Here's how the part is built. I have some questions about the finished solid (model axes, mm). Face numbers are marked on the shaded views. A direction names the side the tool comes from. Give positions to 0.01 mm unless a question says otherwise; leave off trailing zeros. Write each loop counter-clockwise with the first axis right and the second up, starting at its lowest first coordinate (ties: lowest second). Pieces come first, ordered by that corner, then holes. Notation, with made-up numbers: (68, -5.75) -> (83, -5.75) arc R17 cw to (83, 1.25) -> close; hole circle Ø8 at (11, 80). An arc over 180 degrees is marked (long way). Use CSV: the item, a comma, the result in double quotes. Start each with the question number.
(1) For pin 1 Ø1.5 at (x, y) = (12.5, 9.5) entering from -Z; pin 2 Ø5 at (x, z) = (16.8, -5) entering from -Y; pin 3 Ø2.5 at (x, y) = (4.8, 8.6) entering from -Z, each with a flat end and sliding along its axis, tell me the tip position at first contact or that it passes through.
(2) If we mould it in two halves opening along X, with no side actions, what happens to the marked faces 1, 2 and 3? For each: pulls with the +X half, pulls with the -X half, needs draft (parallel to the pull), parting line crosses it, or undercut.
(3) Suppose I cut it at D-D on x = 10.5. List the corners of the cut face in (y, z) for me, plus the area to 3 significant figures.
(4) Suppose I cut it at C-C on x = 4.8. List the corners of the cut face in (y, z) for me, plus the area to 3 significant figures.
(5) I need wall thicknesses on L1, parallel to Y at x = 4.8, z = 1.05; L2, parallel to Z at x = 1.5, y = 9.75; L3, parallel to Z at x = 16.8, y = 13.45. Which ranges of each line are inside material? Lowest first, please. Write a range as [from, to].
(6) Suppose I cut it at B-B on y = 8.6. List the corners of the cut face in (x, z) for me.
(7) Suppose I cut it at A-A on z = -5. List the corners of the cut face in (x, y) for me.
(8) Which directions (+Z, -Z, +X, -X, +Y, -Y) give clear straight access to the entire face, cutting with the end or side of a thin tool? Please do the marked faces 4 and 5.
from build123d import *

# Parameters (mm, degrees)
SKETCH_W     = 19.8
SKETCH_H     = 14.5
SKETCH_R     = 1.5
PAD_DEPTH    = 3
SKETCH001_W  = 19.8
SKETCH001_H  = 3
PAD001_DEPTH = 10
SKETCH002_R  = 1.5
POCKET_DEPTH = 3.001


with BuildPart() as part:
    # Sketch → Pad (new body)
    with BuildSketch(Plane.XY):
        with Locations((9.9, 7.25)):
            Rectangle(SKETCH_W, SKETCH_H)
        with Locations((4.8, 8.6)):
            Circle(SKETCH_R, mode=Mode.SUBTRACT)
        with Locations((15, 8.6)):
            Circle(SKETCH_R, mode=Mode.SUBTRACT)
    extrude(amount=PAD_DEPTH)

    # Sketch001 → Pad001 (new body)
    with BuildSketch(Plane(origin=(0, 0, 0), x_dir=(1, 0, 0), z_dir=(0, 0, -1))):
        with Locations((9.9, -13)):
            Rectangle(SKETCH001_W, SKETCH001_H)
    extrude(amount=PAD001_DEPTH)

    # Sketch002 → Pocket (cut, through all)
    with BuildSketch(Plane.XZ.offset(-11.5)):
        with Locations((3, -5)):
            Circle(SKETCH002_R)
        with Locations((16.8, -5)):
            Circle(SKETCH002_R)
    extrude(amount=-POCKET_DEPTH, mode=Mode.SUBTRACT)


solid = part.part
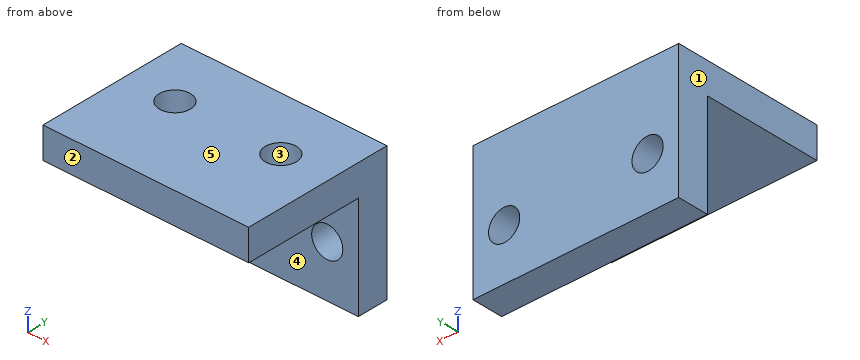
Geometry says:
1,pin 1,"z = 0"
1,pin 2,"y = 11.5"
1,pin 3,"through"
2,face 1,"pulls with the -X half"
2,face 2,"needs draft"
2,face 3,"undercut"
3,outline,"(0, 0) -> (11.5, 0) -> (11.5, -10) -> (14.5, -10) -> (14.5, 3) -> (0, 3) -> close"
3,area,"73.5 mm²"
4,outline,"(0, 0) -> (7.1, 0) -> (7.1, 3) -> (0, 3) -> close; (10.1, 0) -> (11.5, 0) -> (11.5, -10) -> (14.5, -10) -> (14.5, 3) -> (10.1, 3) -> close"
4,area,"64.5 mm²"
5,L1,"[0, 7.1], [10.1, 14.5]"
5,L2,"[0, 3]"
5,L3,"[-10, -6.5], [-3.5, 3]"
6,outline,"(0, 0) -> (3.3, 0) -> (3.3, 3) -> (0, 3) -> close; (6.3, 0) -> (13.5, 0) -> (13.5, 3) -> (6.3, 3) -> close; (16.5, 0) -> (19.8, 0) -> (19.8, 3) -> (16.5, 3) -> close"
7,outline,"(0, 11.5) -> (1.5, 11.5) -> (1.5, 14.5) -> (0, 14.5) -> close; (4.5, 11.5) -> (15.3, 11.5) -> (15.3, 14.5) -> (4.5, 14.5) -> close; (18.3, 11.5) -> (19.8, 11.5) -> (19.8, 14.5) -> (18.3, 14.5) -> close"
8,face 4,"-Z, +X, -X, -Y"
8,face 5,"+Z, +X, -X, +Y, -Y"
